from build123d import *

# Parameters (mm, degrees)
F0_W      = 88
F0_H      = 88
F1_DEPTH  = 1700
F3_DEPTH  = 31
F5_DEPTH  = 31
F7_DEPTH  = 88.001
F9_DEPTH  = 88.001
F11_DEPTH = 31
F13_DEPTH = 31
F14_R     = 5


with BuildPart() as f1:
    # F0 (on Top) → F1 (new body)
    with BuildSketch(Plane.XY):
        with Locations((44, 44)):
            Rectangle(F0_W, F0_H)
    extrude(amount=F1_DEPTH)

    # F2 (on face) → F3 (cut)
    with BuildSketch(Plane.YZ.offset(88)):
        Polygon((29, 282), (44, 282), (59, 282), (59, 370), (29, 370), align=None)
    extrude(amount=-F3_DEPTH, mode=Mode.SUBTRACT)

    # F4 (on face) → F5 (cut)
    with BuildSketch(Plane.YZ.offset(88)):
        Polygon((29, 1460), (44, 1460), (59, 1460), (59, 1548), (29, 1548), align=None)
    extrude(amount=-F5_DEPTH, mode=Mode.SUBTRACT)

    # F6 (on face) → F7 (cut, through all)
    with BuildSketch(Plane.YZ.offset(88)):
        Polygon((0, 1663.5492065112), (88, 1700), (0, 1700), align=None)
    extrude(amount=-F7_DEPTH, mode=Mode.SUBTRACT)

    # F8 (on face) → F9 (cut, through all)
    with BuildSketch(Plane.YZ.offset(88)):
        Polygon((23, 1594.0761184457), (23, 1673.0761184457), (0, 1663.5492065112), (0, 1584.5492065112), align=None)
    extrude(amount=-F9_DEPTH, mode=Mode.SUBTRACT)

    # F10 (on face) → F11 (cut)
    with BuildSketch(Plane(origin=(0, 88, 0), x_dir=(-1, 0, 0), z_dir=(0, 1, 0))):
        Polygon((-59, 162), (-44, 162), (-29, 162), (-29, 250), (-59, 250), align=None)
    extrude(amount=-F11_DEPTH, mode=Mode.SUBTRACT)

    # F12 (on face) → F13 (cut)
    with BuildSketch(Plane(origin=(0, 88, 0), x_dir=(-1, 0, 0), z_dir=(0, 1, 0))):
        Polygon((-59, 1056), (-44, 1056), (-29, 1056), (-29, 1144), (-59, 1144), align=None)
    extrude(amount=-F13_DEPTH, mode=Mode.SUBTRACT)

    # F14
    f14_edges = [f1.edges().sort_by_distance(p)[0] for p in [
        (88, 0, 792.274603),
        (0, 0, 792.274603),
        (88, 88, 850),
        (0, 88, 850),
    ]]
    fillet(f14_edges, radius=F14_R)


solid = f1.part
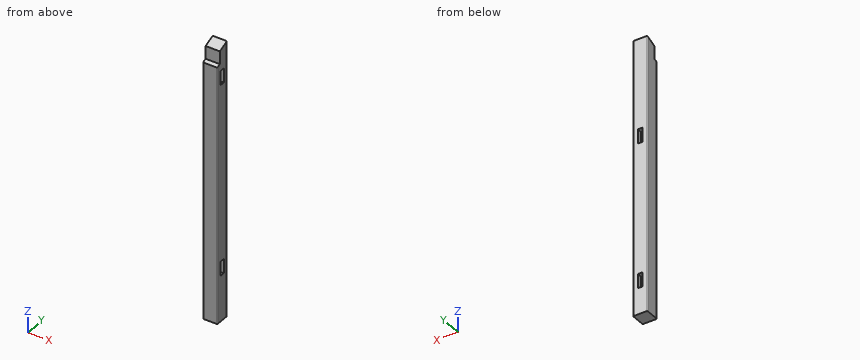
Source: CAD feature listing. Evaluate the final solid. Frame: model axes, mm. Coordinates: 2 decimals unless noted, no trailing zeros. Loops run counter-clockwise (first coordinate to the right, second up) from the corner with the lowest first, then second, coordinate; pieces in that order, holes last. Notation, with made-up numbers: (23.25, 42.25) - (49.25, 42.25) arc R12 ccw to (49.25, 57.25) - close; hole circle Ø10 at (3.25, -8). An arc over 180 degrees is marked (long way). One line per item, written item: value. Start each with the question number.
1. Section B-B (z = 1528). Return the cut outline in (x, y).
2. Contact query for flat-ended pins moving along their axis: P1, Ø9, axis at x = 68, y = 40, coming from the +Z side; P2, Ø15, axis at y = 47.5, z = 330.5, coming from the +X side; P3, Ø5, axis at x = 10.5, y = 69.5, coming from the +Z side. Output: stop coordinate, or through.
3. Ray query, L1, parallel to Z at x = 50, y = 60.5; L2, parallel to Z at x = 77, y = 49; L3, parallel to Z at x = 8, y = 82.5. Return the intervals inside material, ascending.
4. Section A-A (x = 43.5). Return the cut outline in (y, z), and give its area (3 significant figures).
Verdict:
1. outline: (0, 5) arc R5 ccw to (5, 0) - (83, 0) arc R5 ccw to (88, 5) - (88, 29) - (57, 29) - (57, 59) - (88, 59) - (88, 83) arc R5 ccw to (83, 88) - (5, 88) arc R5 ccw to (0, 83) - close
2. P1: stops at z = 1681.98
2. P2: stops at x = 57
2. P3: stops at z = 1693.37
3. L1: z = 0 to 162, 250 to 1056, 1144 to 1688.61
3. L2: z = 0 to 282, 370 to 1460, 1548 to 1683.85
3. L3: z = 0 to 1697.72
4. outline: (0, 0) - (88, 0) - (88, 162) - (57, 162) - (57, 250) - (88, 250) - (88, 1056) - (57, 1056) - (57, 1144) - (88, 1144) - (88, 1700) - (23, 1673.08) - (23, 1594.08) - (0, 1584.55) - close
4. area: 141,000 mm2
